Design review of the part built by this model. Coordinates are the model's own, in mm. A direction names the side the tool comes from. Give positions to 0.01 mm unless a question says otherwise; leave off trailing zeros. Loops run counter-clockwise (first coordinate to the right, second up) from the corner with the lowest first, then second, coordinate; pieces in that order, holes last. Notation, with made-up numbers: M 4,38 L 36,38 A21 ccw 36,75 Z; hole C 78.5,45.5 d7. An arc over 180 degrees is marked long. Use a Markdown table: item, result. Add a question column.
(1) Draft analysis for pull direction Y (two halves, no side actions). For faces 1 (the face through (-9.519, 10, 2)), 2 (the face through (53.57, 22.18, 0.25)), 3 (the face through (26.51, 43.4, 1.82)), state which applies: pulls with the +Y half, pulls with the -Y half, needs draft (parallel to the pull), parting line crosses it, or undercut.
(2) For faces 4 (the face through (78.176, 9.901, 1.565)), 5 (the face through (6, 4.215, 2)), 6 (the face through (61, 23, 0)), 7 (the face through (-8, -0.01, 2)), 8 (the face through (4.981, 1, 2)), list the 3-axis set-ups (+Z, -Z, +X, -X, +Y, -Y) from which the entire face can be reached by the end or side of a thin tool; tool diameter is ignored.
(3) Add section A-A, the plane y = 10. Give the boundary of the cut face in (x, z) (3 decimals).
(4) Add section C-C, the plane z = 1.3. State how many separate pieces and enclosed holes the cut face has, then the cut area to 3 significant figures.
(5) Insertion check: pin 1 Ø0.6 at (y, z) = (31.5, 0.5) entering from -X; pin 2 Ø0.8 at (x, z) = (11.5, 1.5) entering from -Y; pin 3 Ø2.5 at (x, y) = (72.4, 22.4) entering from -Z; pin 4 Ø0.8 at (x, z) = (5.5, 1) entering from +Y. Each pin has a flat end and moves straight along its axis. Give the tip position at first contact, or say it passes through.
(6) Add section B-B, the plane x = 49. Give the boundary of the cut face in (y, z) (3 decimals).
(7) Add section D-D, the plane x = -3.5. Give the boundary of the cut face in (y, z) (3 decimals).
(8) For probe 1 along X at (y, z) = (-1, 2.35); probe 2 along Y at (x, z) = (16, 0.3); probe 3 along X at (y, z) = (8.5, 1.9), list the stretches that pass through material, from the lowest coordinate up.
```python
from build123d import *

# Parameters (mm, degrees)
BOSS_EXTRUDE1_DEPTH = 3.175
SKETCH2_W           = 5
SKETCH2_H           = 3.175
BOSS_EXTRUDE2_DEPTH = 3.175
CUT_EXTRUDE1_DEPTH  = 93.974208943
CUT_EXTRUDE4_DEPTH  = 0.5
CUT_EXTRUDE5_DEPTH  = 93.974208943
SKETCH6_R           = 1.5
CUT_EXTRUDE6_DEPTH  = 93.974208943


with BuildPart() as part:
    # Sketch1 → Boss-Extrude1 (new body)
    with BuildSketch(Plane.XY):
        with BuildLine():
            Line((70.685056323, 37.961813727), (50.215098345, 37.961813727))
            Line((50.215098345, 37.961813727), (27.166207813, 42.019918966))
            Line((27.166207813, 42.019918966), (25.837789145, 44.817651071))
            Line((25.837789145, 44.817651071), (-9.51883745, 44.817651071))
            Line((-9.51883745, 44.817651071), (-9.51883745, -0.009767361))
            Line((-9.51883745, -0.009767361), (25.837789145, -0.009767361))
            Line((25.837789145, -0.009767361), (27.166207813, 2.787964744))
            Line((27.166207813, 2.787964744), (50.215098345, 6.846069984))
            Line((50.215098345, 6.846069984), (70.685056323, 6.846069984))
            ThreePointArc((70.685056323, 6.846069984), (78.259672242, 9.983578627), (81.397180885, 17.558194546))
            Line((81.397180885, 17.558194546), (81.397180885, 22.403941855))
            Line((81.397180885, 22.403941855), (81.397180885, 27.249689164))
            ThreePointArc((81.397180885, 27.249689164), (78.259672242, 34.824305083), (70.685056323, 37.961813727))
        make_face()
    extrude(amount=BOSS_EXTRUDE1_DEPTH)

    # Sketch2 → Boss-Extrude2 (add)
    with BuildSketch(Plane.XY.offset(3.175)):
        with Locations((-4.01883745, -1.597267361)):
            Rectangle(SKETCH2_W, SKETCH2_H)
        with Locations((20.98116255, -1.597267361)):
            Rectangle(SKETCH2_W, SKETCH2_H)
    extrude(amount=-BOSS_EXTRUDE2_DEPTH)

    # Sketch3 → Cut-Extrude1 (cut, through all)
    with BuildSketch(Plane.XY.offset(3.175)):
        Polygon((4.98116255, -0.009767361), (1.98116255, -0.009767361), (1.98116255, 1.815232639), (0.43116255, 1.815232639), (0.43116255, 4.215232639), (1.98116255, 4.215232639), (1.98116255, 8.815232639), (4.98116255, 8.815232639), (4.98116255, 4.215232639), (6.53116255, 4.215232639), (6.53116255, 1.815232639), (4.98116255, 1.815232639), align=None)
        Polygon((11.98116255, -0.009767361), (11.98116255, 1.815232639), (10.43116255, 1.815232639), (10.43116255, 4.215232639), (11.98116255, 4.215232639), (11.98116255, 8.815232639), (14.98116255, 8.815232639), (14.98116255, 4.215232639), (16.53116255, 4.215232639), (16.53116255, 1.815232639), (14.98116255, 1.815232639), (14.98116255, -0.009767361), align=None)
    extrude(amount=-CUT_EXTRUDE1_DEPTH, mode=Mode.SUBTRACT)

    # Sketch4 → Cut-Extrude4 (cut)
    with BuildSketch(Plane.XY):
        Polygon((25.837789145, 22.403941855), (27.166207813, 22.403941855), (27.166207813, 42.019918966), (25.837789145, 44.817651071), align=None)
        Polygon((27.166207813, 2.787964744), (27.166207813, 22.403941855), (25.837789145, 22.403941855), (25.837789145, -0.009767361), align=None)
        with BuildLine():
            Line((50.215098345, 6.846069984), (51.495792338, 6.846069984))
            ThreePointArc((51.495792338, 6.846069984), (53.570887609, 22.403941855), (51.495792338, 37.961813727))
            Line((51.495792338, 37.961813727), (50.215098345, 37.961813727))
            ThreePointArc((50.215098345, 37.961813727), (52.343297045, 22.403941855), (50.215098345, 6.846069984))
        make_face()
        with BuildLine():
            Line((70.685056323, 37.961813727), (70.685056323, 6.846069984))
            ThreePointArc((70.685056323, 6.846069984), (71.126055593, 6.855151414), (71.56630713, 6.882380308))
            Line((71.56630713, 6.882380308), (71.56630713, 37.925503403))
            ThreePointArc((71.56630713, 37.925503403), (71.126055593, 37.952732296), (70.685056323, 37.961813727))
        make_face()
    extrude(amount=CUT_EXTRUDE4_DEPTH, mode=Mode.SUBTRACT)

    # Sketch5 → Cut-Extrude5 (cut, through all)
    with BuildSketch(Plane.XY.offset(3.175)):
        with BuildLine():
            Line((15.48116255, 44.817651071), (-9.51883745, 44.817651071))
            Line((-9.51883745, 44.817651071), (-9.51883745, 19.817651071))
            ThreePointArc((-9.51883745, 19.817651071), (-2.196506979, 37.495320601), (15.48116255, 44.817651071))
        make_face()
    extrude(amount=-CUT_EXTRUDE5_DEPTH, mode=Mode.SUBTRACT)

    # Sketch6 → Cut-Extrude6 (cut, through all)
    with BuildSketch(Plane.XY.offset(3.175)):
        with Locations((78.397180885, 22.403941855)):
            Circle(SKETCH6_R)
        with Locations((72.397180885, 22.403941855)):
            Circle(SKETCH6_R)
    extrude(amount=-CUT_EXTRUDE6_DEPTH, mode=Mode.SUBTRACT)


solid = part.part
```
Established:
| question | item | result |
|---|---|---|
| 1 | face 1 | needs draft |
| 1 | face 2 | undercut |
| 1 | face 3 | pulls with the +Y half |
| 2 | face 4 | +Z, -Z, +X, -Y |
| 2 | face 5 | +Z, -Z |
| 2 | face 6 | -Z, +X, -X, +Y, -Y |
| 2 | face 7 | +Z, -Z, -X, -Y |
| 2 | face 8 | +Z, -Z, -Y |
| 3 | outline | M -9.519,0 L 25.838,0 L 25.838,0.5 L 27.166,0.5 L 27.166,0 L 51,0 L 51,0.5 L 52.26,0.5 L 52.26,0 L 70.685,0 L 70.685,0.5 L 71.566,0.5 L 71.566,0 L 78.276,0 L 78.276,3.175 L -9.519,3.175 Z |
| 4 | separate pieces | 1 |
| 4 | enclosed holes | 2 |
| 4 | area | 3,190 mm^2 |
| 5 | pin 1 | x = -6.78 |
| 5 | pin 2 | y = -0.01 |
| 5 | pin 3 | through |
| 5 | pin 4 | y = 42.91 |
| 6 | outline | M 6.632,0 L 38.176,0 L 38.176,3.175 L 6.632,3.175 Z |
| 7 | outline | M -3.185,0 L 36.088,0 L 36.088,3.175 L -3.185,3.175 Z |
| 8 | probe 1 | -6.52 to -1.52, 18.48 to 23.48 |
| 8 | probe 2 | -0.01 to 1.82, 4.22 to 44.82 |
| 8 | probe 3 | -9.52 to 1.98, 4.98 to 11.98, 14.98 to 76.4 |
